Source: CAD feature listing. Evaluate the final solid. Frame: model axes, mm. Face numbers are marked on the shaded views. A direction names the side the tool comes from. Round coordinates to 2 decimals unless told otherwise and drop trailing zeros. Loops run counter-clockwise (first coordinate to the right, second up) from the corner with the lowest first, then second, coordinate; pieces in that order, holes last.
Item 1: Section query C-C on x = -54. Return loops of the section in (y, z), then the cut area to 3 significant figures.
Item 2: Ray query, L1, parallel to Y at x = 0, z = 280; L2, parallel to Y at x = -34, z = -50; L3, parallel to Z at x = -7, y = -15.5. Return the intervals inside material, ascending.
Item 3: Section query B-B on z = -50. Return loops of the section in (x, y).
Item 4: Access query for the marked faces 1 and 2. Directions: +Z, -Z, +X, -X, +Y, -Y. A direction counts if a zero-diameter tool reaches every point of the face in a straight line with its end or side. Return the directions, or none.
Item 5: Section query D-D on z = 397. Return loops of the section in (x, y).
Item 6: Section query A-A on y = 0. Return loops of the section in (x, z).
Item 7: First-contact query: P1, Ø1.5, axis at x = -44, y = 18, coming from the +Z side; P2, Ø2, axis at x = -17.5, z = 359, coming from the -Y side; P3, Ø10, axis at y = 25, z = 337.5, coming from the -X side. Flat tips, straight axial feed; report the tip coordinate or a pass-through.
```python
from build123d import *

# Parameters (mm, degrees)
IZIM1_R                     = 45
Y_KSEKLIK_EKSTR_ZYON1_DEPTH = 725
IZIM2_R                     = 35
KES_EKSTR_ZYON1_DEPTH       = 600
IZIM3_R                     = 30
Y_KSEKLIK_EKSTR_ZYON2_DEPTH = 90


with BuildPart() as part:
    # Çizim1 → Yükseklik-Ekstrüzyon1 (new body)
    with BuildSketch(Plane.XY):
        Circle(IZIM1_R)
    extrude(amount=Y_KSEKLIK_EKSTR_ZYON1_DEPTH)

    # Çizim2 → Kes-Ekstrüzyon1 (cut)
    with BuildSketch(Plane.XY.offset(725)):
        Circle(IZIM2_R)
    extrude(amount=-KES_EKSTR_ZYON1_DEPTH, mode=Mode.SUBTRACT)

    # Çizim3 → Yükseklik-Ekstrüzyon2 (add, symmetric)
    with BuildSketch(Plane(origin=(0, 0, 0), x_dir=(0, 0, -1), z_dir=(1, 0, 0))):
        with BuildLine():
            Line((0, 10), (11.270166538, 10))
            ThreePointArc((11.270166538, 10), (90, 0), (11.270166538, -10))
            Line((11.270166538, -10), (0, -10))
            Line((0, -10), (0, 10))
        make_face()
        with Locations(Location((50, 0, 0), (0, 0, 180))):
            Circle(IZIM3_R, mode=Mode.SUBTRACT)
    extrude(amount=Y_KSEKLIK_EKSTR_ZYON2_DEPTH, both=True)


solid = part.part
```
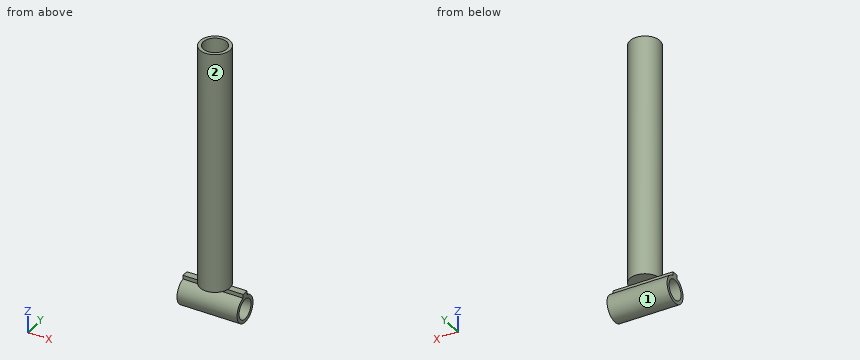
Data:
1. outline: (-10, -11.27) arc R40 ccw (long way) to (10, -11.27) - (10, 0) - (-10, 0) - close; hole circle Ø60 at (0, -50)
1. area: 2,410 mm2
2. L1: y = -45 to -35, 35 to 45
2. L2: y = -40 to -30, 30 to 40
2. L3: z = -86.87 to -75.69, -24.31 to -13.13, 0 to 125
3. outline: (-90, -40) - (90, -40) - (90, -30) - (-90, -30) - close; (-90, 30) - (90, 30) - (90, 40) - (-90, 40) - close
4. face 1: +X, -X
4. face 2: +Z
5. outline: circle Ø90 at (0, 0); hole circle Ø70 at (0, 0)
6. outline: (-90, -90) - (90, -90) - (90, -80) - (-90, -80) - close; (-90, -20) - (90, -20) - (90, 0) - (45, 0) - (45, 725) - (35, 725) - (35, 125) - (-35, 125) - (-35, 725) - (-45, 725) - (-45, 0) - (-90, 0) - close
7. P1: stops at z = -13.91
7. P2: stops at y = -41.87
7. P3: stops at x = -40.31
